Autodesk Inventor part; units mm, degrees
ref_plane "YZ Plane" through (0, 0, 0) normal (1, 0, 0) x (0, 1, 0)
ref_plane "XZ Plane" through (0, 0, 0) normal (0, 1, 0) x (-1, 0, 0)
ref_plane "XY Plane" through (0, 0, 0) normal (0, 0, 1) x (1, 0, 0)
sketch "Sketch1" plane through (0, 0, 0) normal (0, 1, 0) x (-1, 0, 0)
  line L0 (0, 0) -> (0, 6.5)
  line L1 (0, 0) -> (20, 0)
  line L2 (-2, -2) -> (20, -2)
  line L3 (-2, 0) -> (-2, 6.5)
  line L4 (20, -2) -> (20, 0)
  line L5 (-2, 0) -> (-8.5, 0)
  line L6 (-8.5, -2) -> (-2, -2)
  line L7 (-8.5, 0) -> (-8.5, -2)
  line L8 (-2, 6.5) -> (0, 6.5)
  dimension "d2" = 20
  dimension "d3" = 2
  dimension "d5" = 2
  dimension "d30" = 6.5
  dimension "d33" = 6.5
extrude "Extrusion1" add sketch "Sketch1" along normal blind 40
sketch "Sketch2" plane through (0, 0, 0) normal (0, -1, 0) x (1, 0, 0)
  line L0 (2, 0) -> (8.5, 0)
  line L1 (8.5, 0) -> (8.5, 6.5)
  line L2 (8.5, 6.5) -> (2, 6.5)
  line L3 (2, 6.5) -> (2, 0)
  point P0 (0, 0)
  dimension "d10" = 6.5
  dimension "d11" = 6.5
extrude "Extrusion2" add sketch "Sketch2" against normal blind 10
sketch "Sketch3" plane through (22, 0, -2) normal (0, 0, -1) x (-1, 0, 0)
  line L0 (42, 0) -> (42, 40)
  circle A0 centre (32, 20) radius 3.5
  circle A1 centre (32, 20) radius 2
  line L1 (32, 20) -> (42, 20)
  line L2 (42, 0) -> (42, 40)
  point P0 (22, 0)
  dimension "d15" = 7
  dimension "d18" = 4
  dimension "d32" = 10
hole "Hole1" at (-10, 20, -2) direction (0, 0, 1) diameter 4 end through all countersink diameter 7 countersink angle 90
properties part number "3DPrintBracket" material "PC/ABS Plastic"
Could you check a few things on this model? Use its own coordinates, in mm. A direction names the side the tool comes from. Coordinates: 2 decimals unless noted, no trailing zeros. Order: outer loops, then holes, each group sorted by start corner. A loop starts at its lowest first (then second) coordinate and runs counter-clockwise, first axis right, second up. Notation, with made-up numbers: (42.5, 69) -> (62.5, 69) arc R16 cw to (62.5, 78) -> close; hole circle Ø8 at (62.5, -23.5). An arc over 180 degrees is marked (long way). One line per item, written item: value. Start each with the question number.
1) Which directions (+Z, -Z, +X, -X, +Y, -Y) give clear straight access to the entire face, cutting with the end or side of a thin tool? Please do faces 1 (the flat face through (-7.6, 19.7, 0)), 2 (the flat face through (8.5, 11, -1)), 3 (the flat face through (5, 25, 0)).
2) I'm going to push flat-ended pins straight in: pin 1 (3 mm diameter, centred on y = 26, z = 3, fed in from +X); pin 2 (1 mm diameter, centred on y = 8, z = 3.5, fed in from -X); pin 3 (4 mm diameter, centred on x = -4, y = 33.5, fed in from +Z). Where does each tip first touch, or does it pass through?
3) Imagine slicing it at C-C on y = 34.5. List the corners of the cut face in (x, z) for me.
4) We'd pull the mould along X, two halves only. Please class faces 4 (the flat face through (0, 20, 3)), 5 (the flat face through (1, 11, 6.5)), 6 (the cylindrical face through (-11.352, 18.526, -0.246)): +X half, -X half, draft (parallel to the pull), parting line (faces both ways), or undercut.
5) If I drill on L1, parallel to Y at x = -10, z = -0.2; L2, parallel to X at y = 20, z = -0.15; L3, parallel to X at y = 28.5, z = 5.75, over which ranges is the centre line in solid material (lowest first)? Write a range as [from, to].
6) Imagine slicing it at B-B on y = 20. List the corners of the cut face in (x, z) for me, plus the area to 4 significant figures.
7) Imagine slicing it at D-D on z = 2.25. List the corners of the cut face in (x, y) for me, plus the area to 3 significant figures.
8) Imagine slicing it at A-A on x = -10. List the corners of the cut face in (y, z) for me.
Answer list:
1. face 1: +Z, -X, +Y, -Y
1. face 2: +Z, -Z, +X, +Y, -Y
1. face 3: +Z, +X, +Y
2. pin 1: stops at x = 2
2. pin 2: stops at x = 0
2. pin 3: stops at z = 0
3. outline: (-20, -2) -> (8.5, -2) -> (8.5, 0) -> (2, 0) -> (2, 6.5) -> (0, 6.5) -> (0, 0) -> (-20, 0) -> close
4. face 4: -X half
4. face 5: draft
4. face 6: undercut
5. L1: y = [0, 18], [22, 40]
5. L2: x = [-20, -12], [-8, 8.5]
5. L3: x = [0, 2]
6. outline: (-20, -2) -> (-13.5, -2) -> (-12, -0.5) -> (-12, 0) -> (-20, 0) -> close; (-8, -0.5) -> (-6.5, -2) -> (8.5, -2) -> (8.5, 0) -> (2, 0) -> (2, 6.5) -> (0, 6.5) -> (0, 0) -> (-8, 0) -> close
6. area: 59.75 mm2
7. outline: (0, 0) -> (8.5, 0) -> (8.5, 10) -> (2, 10) -> (2, 40) -> (0, 40) -> close
7. area: 145 mm2
8. outline: (0, -2) -> (16.5, -2) -> (18, -0.5) -> (18, 0) -> (0, 0) -> close; (22, -0.5) -> (23.5, -2) -> (40, -2) -> (40, 0) -> (22, 0) -> close
